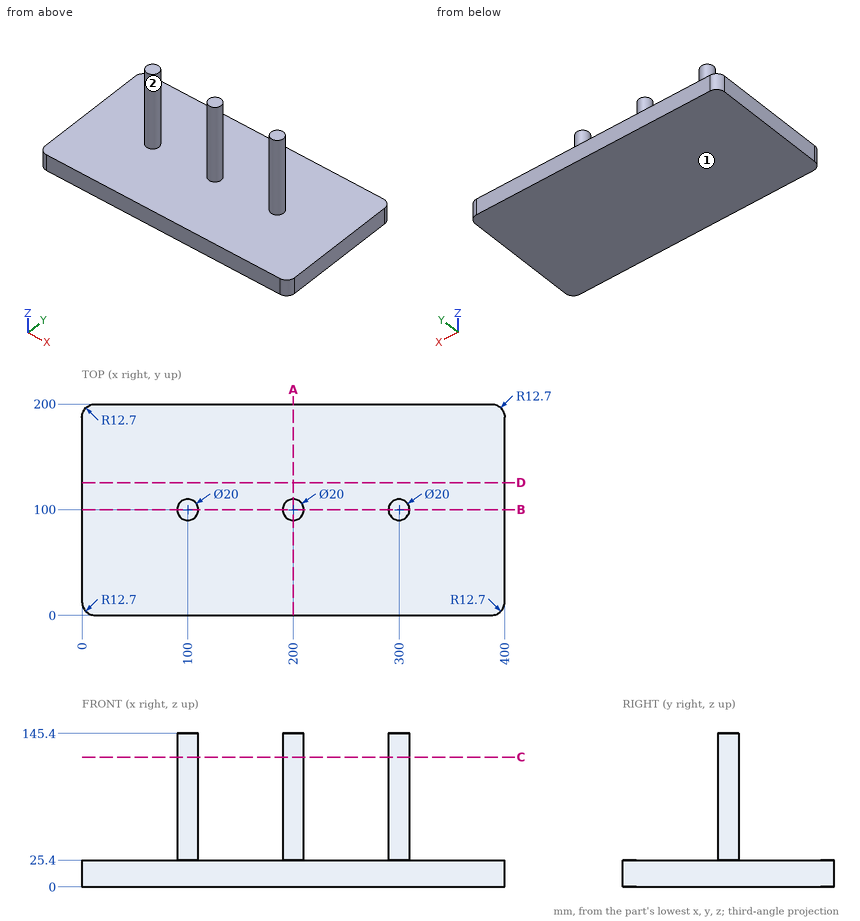
Study the drawing (mm; zero at the part's minimum x, y, z) and answer. Round coordinates to 2 decimals unless told otherwise and drop trailing zeros. Write each loop counter-clockwise with the first axis right and the second up, starting at its lowest first coordinate (ties: lowest second). Pieces come first, ordered by that corner, then holes. Notation, with made-up numbers: (66, -21) - (72, -21) arc R20 ccw to (72, -7) - close; hole circle Ø1 at (12.5, -35). An arc over 180 degrees is marked (long way). Use a Markdown table: item, result. Add a question column.
1. Flat-ended cylindrical pins translate along their axes: P1, Ø6, axis at x = 319, y = 33.5, coming from the +Z side; P2, Ø3, axis at x = 46.5, z = 28, coming from the +Y side; P3, Ø6, axis at x = 315.5, y = 76, coming from the -Z side. Find the tip coordinate at first contact, or state that the pin passes through.
2. Consider line 1 (Z direction, x = 39.5, y = 103); line 2 (X direction, y = 92.5, z = 98.5); line 3 (Y direction, x = 199.5, z = 61). Determine where each line is inside the solid, lowest interval first.
3. The part is cut by section B-B (y = 100). Write down the section's boundary in (x, z).
4. The part is cut by section D-D (y = 125.5). Write down the section's boundary in (x, z), and give its area (3 significant figures).
5. The part is cut by section A-A (x = 200). Write down the section's boundary in (y, z).
6. For a pull along X with two mould halves and no side action, classify the marked faces 1 and 2 as +X half, -X half, draft (parallel to the pull), parting line (faces both ways), or undercut.
7. The part is cut by section C-C (z = 123). Write down the section's boundary in (x, y), and give its area (3 significant figures).
Reported:
| question | item | result |
|---|---|---|
| 1 | P1 | z = 25.4 |
| 1 | P2 | through |
| 1 | P3 | z = 0 |
| 2 | line 1 | 0 to 25.4 |
| 2 | line 2 | 93.39 to 106.61, 193.39 to 206.61, 293.39 to 306.61 |
| 2 | line 3 | 90.01 to 109.99 |
| 3 | outline | (0, 0) - (400, 0) - (400, 25.4) - (310, 25.4) - (310, 145.4) - (290, 145.4) - (290, 25.4) - (210, 25.4) - (210, 145.4) - (190, 145.4) - (190, 25.4) - (110, 25.4) - (110, 145.4) - (90, 145.4) - (90, 25.4) - (0, 25.4) - close |
| 4 | outline | (0, 0) - (400, 0) - (400, 25.4) - (0, 25.4) - close |
| 4 | area | 10,200 mm^2 |
| 5 | outline | (0, 0) - (200, 0) - (200, 25.4) - (110, 25.4) - (110, 145.4) - (90, 145.4) - (90, 25.4) - (0, 25.4) - close |
| 6 | face 1 | draft |
| 6 | face 2 | undercut |
| 7 | outline | circle Ø20 at (100, 100); circle Ø20 at (200, 100); circle Ø20 at (300, 100) |
| 7 | area | 942 mm^2 |
